from build123d import *

# Parameters (mm, degrees)
SKETCH1_R           = 31.75
SKETCH1_R_2         = 1.65
BOSS_EXTRUDE1_DEPTH = 3
SKETCH2_W           = 9
SKETCH2_H           = 10
SKETCH2_W_2         = 5
SKETCH2_H_2         = 6
BOSS_EXTRUDE2_DEPTH = 10


with BuildPart() as part:
    # Sketch1 → Boss-Extrude1 (new body)
    with BuildSketch(Plane(origin=(0, 0, 0), x_dir=(1, 0, 0), z_dir=(0, 1, 0))):
        with Locations(Location((0, 0, 0), (0, 0, 270))):
            Circle(SKETCH1_R)
        with Locations(Location((4.08, 2.5, 0), (0, 0, 270))):
            Circle(SKETCH1_R_2, mode=Mode.SUBTRACT)
        with Locations(Location((4.08, -2.5, 0), (0, 0, 270))):
            Circle(SKETCH1_R_2, mode=Mode.SUBTRACT)
    extrude(amount=BOSS_EXTRUDE1_DEPTH)

    # Sketch2 → Boss-Extrude2 (add)
    # profile 1 of 2: a face of its own
    with BuildSketch(Plane(origin=(0, 3, 0), x_dir=(1, 0, 0), z_dir=(0, 1, 0))):
        with Locations((12.875, 0)):
            Rectangle(SKETCH2_W, SKETCH2_H)
        with Locations((12.875, 0)):
            Rectangle(SKETCH2_W_2, SKETCH2_H_2, mode=Mode.SUBTRACT)
    # profile 2 of 2: a face of its own
    with BuildSketch(Plane(origin=(0, 3, 0), x_dir=(1, 0, 0), z_dir=(0, 1, 0))):
        with Locations((-12.875, 0)):
            Rectangle(SKETCH2_W, SKETCH2_H)
        with Locations((-12.875, 0)):
            Rectangle(SKETCH2_W_2, SKETCH2_H_2, mode=Mode.SUBTRACT)
    extrude(amount=BOSS_EXTRUDE2_DEPTH)


solid = part.part
Check sheet for the modelled part. Datum: model origin and axes. Units: mm. A direction names the side the tool comes from. Give positions to 0.01 mm unless a question says otherwise; leave off trailing zeros. Loops run counter-clockwise (first coordinate to the right, second up) from the corner with the lowest first, then second, coordinate; pieces in that order, holes last. Notation, with made-up numbers: M 17.25,-32.5 L 45.25,-32.5 A19 ccw 45.25,3.5 Z; hole C -25,-18.5 d11. An arc over 180 degrees is marked long. Use a Markdown table: item, result. Add a question column.
Q1. Go/stop test with flat-tipped pins: pin 1 (4 mm diameter, centred on x = 9, y = 7, fed in from +Z); pin 2 (1.8 mm diameter, centred on y = 6.5, z = 0.5, fed in from -X) (3 decimals); pin 3 (1.8 mm diameter, centred on y = 10, z = 0.5, fed in from +X) (3 decimals). Record where each tip stops, or that it passes through.
Q2. Tool access check on faces 1 (the flat face through (13, 8, 5)), 2 (the flat face through (-13, 3, 0)), 3 (the flat face through (13, 8, -5)), 4 (the cylindrical face through (4.576, 1.479, -0.926)). Record the directions out of +Z, -Z, +X, -X, +Y, -Y that give a thin tool (end or side, any length) a straight path to the whole face; none if there is none.
Q3. Sectioned sample at C-C, the plane z = 0. Record the cut outline in (x, y) (3 decimals), then the cut area to 4 significant figures.
Q4. Mould release check, pull along X, two halves, no side actions. Record for faces 5 (the flat face through (-17.375, 8, 0)), 6 (the flat face through (17.375, 8, 0)), 7 (the flat face through (-13, 8, -3)), 8 (the flat face through (-10, 13, 0)): pulls with the +X half, pulls with the -X half, needs draft (parallel to the pull), parting line crosses it, or undercut.
Q5. Scan lines: line 1 along Z through (x, y) = (12.5, 4.5); line 2 along Y through (x, z) = (1, 19); line 3 along X through (y, z) = (2.25, -2.5). Record each from-to range of solid material in increasing order. Write a range as [from, to].
Q6. Sectioned sample at D-D, the plane x = -13. Record the cut outline in (y, z).
Q7. Sectioned sample at B-B, the plane x = 4.08. Record the cut outline in (y, z), then the cut area to 3 significant figures.
Q8. Sectioned sample at A-A, the plane y = 5.5. Record the cut outline in (x, z) (3 decimals).
Verdict:
| question | item | result |
|---|---|---|
| 1 | pin 1 | z = 5 |
| 1 | pin 2 | x = -17.375 |
| 1 | pin 3 | x = 17.375 |
| 2 | face 1 | +Z, +X, -X, +Y |
| 2 | face 2 | +Y |
| 2 | face 3 | -Z, +X, -X, +Y |
| 2 | face 4 | +Y, -Y |
| 3 | outline | M -31.75,0 L 31.75,0 L 31.75,3 L 17.375,3 L 17.375,13 L 15.375,13 L 15.375,3 L 10.375,3 L 10.375,13 L 8.375,13 L 8.375,3 L -8.375,3 L -8.375,13 L -10.375,13 L -10.375,3 L -15.375,3 L -15.375,13 L -17.375,13 L -17.375,3 L -31.75,3 Z |
| 3 | area | 270.5 mm^2 |
| 4 | face 5 | pulls with the -X half |
| 4 | face 6 | pulls with the +X half |
| 4 | face 7 | undercut |
| 4 | face 8 | needs draft |
| 5 | line 1 | [-5, -3], [3, 5] |
| 5 | line 2 | [0, 3] |
| 5 | line 3 | [-31.65, 2.43], [5.73, 31.65] |
| 6 | outline | M 0,-28.97 L 3,-28.97 L 3,-5 L 13,-5 L 13,-3 L 3,-3 L 3,3 L 13,3 L 13,5 L 3,5 L 3,28.97 L 0,28.97 Z |
| 7 | outline | M 0,-31.49 L 3,-31.49 L 3,-4.15 L 0,-4.15 Z; M 0,-0.85 L 3,-0.85 L 3,0.85 L 0,0.85 Z; M 0,4.15 L 3,4.15 L 3,31.49 L 0,31.49 Z |
| 7 | area | 169 mm^2 |
| 8 | outline | M -17.375,-5 L -8.375,-5 L -8.375,5 L -17.375,5 Z; M 8.375,-5 L 17.375,-5 L 17.375,5 L 8.375,5 Z; hole M -15.375,-3 L -10.375,-3 L -10.375,3 L -15.375,3 Z; hole M 10.375,-3 L 15.375,-3 L 15.375,3 L 10.375,3 Z |
